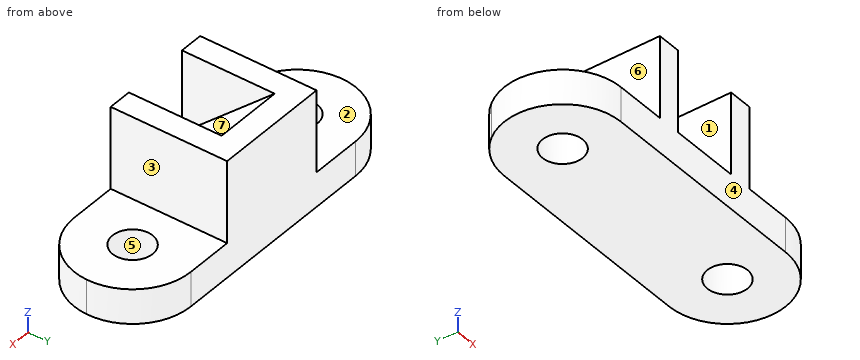
Autodesk Fusion 360 part; units mm, degrees
sketch "Sketch1" plane through (0, 0, 0) normal (0, 0, 1) x (1, 0, 0)
  line L0 (28.0323, 19.5121) -> (146.0361, 19.5121)
  line L1 (178.0242, -13.3588) -> (178.0327, -13.3589)
  line L2 (146.0457, -44.448) -> (28.0654, -44.448)
  line L3 (2.8649, 7.2735) -> (2.8643, 7.275)
  arc A0 (2.8649, 7.2735) -> (28.0654, -44.448) centre (28.0654, -12.448) ccw
  arc A1 (28.0323, 19.5121) -> (2.8643, 7.275) centre (28.0323, -12.4879) ccw
  arc A2 (178.0242, -13.3588) -> (146.0361, 19.5121) centre (146.0361, -12.4879) ccw
  arc A3 (146.0457, -44.448) -> (178.0327, -13.3589) centre (146.0457, -12.448) ccw
  circle A4 centre (28, -12.5) radius 11
  circle A5 centre (146, -12.5) radius 11
  line L4 (55.9792, 19.5121) -> (119.9792, 19.5121)
  line L5 (119.9792, 19.5121) -> (119.9792, -44.4879)
  line L6 (119.9792, -44.4879) -> (55.9792, -44.4879)
  line L7 (55.9792, -44.4879) -> (55.9792, 19.5121)
  point P0 (-1.9465, 19.5121)
  point P1 (176.0535, 19.5121)
  point P2 (0.3124, -44.448)
  dimension "d1" = 178
  dimension "d2" = 64
  dimension "d3" = 32
  dimension "d4" = 32
  dimension "d5" = 32
  dimension "d6" = 32
  dimension "d7" = 22
  dimension "d8" = 22
  dimension "d9" = 64
  dimension "d10" = 64
extrude "Extrude1" add sketch "Sketch1" along normal blind 19 contours L0 L2 A0 A1 L7 | L0 L2 L4 L5 L7 | L0 L1 L2 A2 A3 L5
sketch "Sketch2" plane through (0, 0, 19) normal (0, 0, 1) x (-1, 0, 0)
  circle A0 centre (-146, 12.5) radius 11
  circle A1 centre (-28, 12.5) radius 11
  arc A2 (-28.0323, -19.5121) -> (-2.8643, -7.275) centre (-28.0323, 12.4879) ccw
  line L0 (-2.8643, -7.275) -> (-2.8649, -7.2735)
  arc A3 (-2.8649, -7.2735) -> (-28.0654, 44.448) centre (-28.0654, 12.448) ccw
  line L1 (-28.0654, 44.448) -> (-146.0457, 44.448)
  arc A4 (-146.0457, 44.448) -> (-178.0327, 13.3589) centre (-146.0457, 12.448) ccw
  line L2 (-178.0327, 13.3589) -> (-178.0242, 13.3588)
  arc A5 (-178.0242, 13.3588) -> (-146.0361, -19.5121) centre (-146.0361, 12.4879) ccw
  line L3 (-146.0361, -19.5121) -> (-28.0323, -19.5121)
  line L4 (-56.0201, -19.5121) -> (-120.0201, -19.5121)
  line L5 (-120.0201, -19.5121) -> (-120.0201, 44.4879)
  line L6 (-120.0201, 44.4879) -> (-56.0201, 44.4879)
  line L7 (-56.0201, 44.4879) -> (-56.0201, -19.5121)
  line L8 (-56.0201, 44.4879) -> (-69.0201, 44.4879)
  line L9 (-69.0201, 44.4879) -> (-69.0201, -6.5121)
  line L10 (-69.0201, -6.5121) -> (-107.0201, -6.5121)
  line L11 (-107.0201, -6.5121) -> (-107.0201, 44.4879)
  line L12 (-107.0201, 44.4879) -> (-120.0201, 44.4879)
  dimension "d13" = 64
  dimension "d14" = 64
  dimension "d15" = 13
  dimension "d16" = 51
  dimension "d17" = 38
  dimension "d18" = 51
extrude "Extrude2" add sketch "Sketch2" along normal blind 45 contours L1 L3 L4 L5 L7 L9 L10 L11
sketch "Sketch3" plane through (69.0201, 0, 0) normal (1, 0, 0) x (0, 1, 0)
  line L0 (-44.448, 19) -> (6.5121, 19)
  line L1 (6.5121, 19) -> (6.5121, 64)
  line L2 (6.5121, 64) -> (-44.448, 64)
  line L3 (-44.448, 64) -> (-44.448, 19)
  line L4 (-44.448, 19) -> (6.552, 19)
  line L5 (6.552, 19) -> (6.5121, 64)
  line L6 (6.5121, 64) -> (-44.448, 19)
  dimension "d21" = 51
extrude "Extrude3" add sketch "Sketch3" along normal blind 38 contours L0 L1 L4 L6
Model file for the job. Use its own axes, mm. Face numbers are marked on the shaded views. A direction names the side the tool comes from. Coordinates: 2 decimals unless noted, no trailing zeros. Order: outer loops, then holes, each group sorted by start corner. A loop starts at its lowest first (then second) coordinate and runs counter-clockwise, first axis right, second up. Notation, with made-up numbers: M 56.25,84 L 66.25,84 A17 ccw 66.25,117 Z; hole C -39.5,-25 d3. An arc over 180 degrees is marked long. Return JSON: item names as keys, results as strings.
1. Tool access for the marked faces 1, 2, 3 and 4: list every direction of +Z, -Z, +X, -X, +Y, -Y with a clear straight run to the whole face (end or side of a thin tool).
Ans:
{"face 1": "+Z, -Y", "face 2": "+Z, -X, +Y, -Y", "face 3": "+Z, +X, +Y, -Y", "face 4": "+Z, -Z, +X, -X, -Y"}
2. Saw through at B-B (x = 148.5). Give the cut face in (y, z), and give its area (3 significant figures).
Ans:
{"outline": "M -44.35,0 L -23.21,0 L -23.21,19 L -44.35,19 Z; M -1.79,0 L 19.42,0 L 19.42,19 L -1.79,19 Z", "area": "805 mm^2"}
3. Saw through at A-A (z = 14.5). Give the number of separate pieces and of enclosed holes in the cut face, and give its area (3 significant figures).
Ans:
{"separate pieces": "1", "enclosed holes": "2", "area": "10,000 mm^2"}
4. Saw through at C-C (y = -19.5). Give the cut face in (x, z), and give its area (3 significant figures).
Ans:
{"outline": "M -3.15,0 L 19.51,0 L 19.51,19 L -3.15,19 Z; M 36.49,0 L 137.51,0 L 137.51,19 L 120.02,19 L 120.02,64 L 107.02,64 L 107.02,41.03 L 69.02,41.03 L 69.02,64 L 56.02,64 L 56.02,19 L 36.49,19 Z; M 154.49,0 L 177.26,0 L 177.26,19 L 154.49,19 Z", "area": "4,790 mm^2"}
5. Flat gauge pins, fed straight in: pin 1 (8 mm diameter, centred on y = -18, z = 30, fed in from -X); pin 2 (13.5 mm diameter, centred on y = -18.5, z = 33, fed in from +X); pin 3 (17.5 mm diameter, centred on x = 156, y = -26, fed in from +Z). Where does each tip first touch, or does it go through?
Ans:
{"pin 1": "x = 56.02", "pin 2": "x = 120.02", "pin 3": "z = 19"}
6. Pull direction Y, two halves, no side cores. Call the marked faces 5, 6 and 7: +Y half, -Y half, draft (parallel to the pull), parting line (faces both ways), or undercut.
Ans:
{"face 5": "undercut", "face 6": "draft", "face 7": "-Y half"}
7. Drill centre lines: probe 1 along X at (y, z) = (-12, 14); probe 2 along Y at (x, z) = (146, 11); probe 3 along X at (y, z) = (-32, 40.5). Where is each one in solid material? Low to high.
Ans:
{"probe 1": "-3.93 to 17.01, 38.99 to 135.01, 156.99 to 178.03", "probe 2": "-44.45 to -23.5, -1.5 to 19.51", "probe 3": "56.02 to 69.02, 107.02 to 120.02"}
8. Saw through at D-D (z = 44). Give the cut face in (x, y).
Ans:
{"outline": "M 56.02,-44.45 L 69.02,-44.45 L 69.02,-16.14 L 107.02,-16.14 L 107.02,-44.45 L 120.02,-44.45 L 120.02,19.51 L 56.02,19.51 Z"}
